Geometry: final body of the model. Coordinates: model frame, mm. Face numbers are marked on the shaded views. A direction names the side the tool comes from. Give positions to 0.01 mm unless a question says otherwise; leave off trailing zeros. Loops run counter-clockwise (first coordinate to the right, second up) from the corner with the lowest first, then second, coordinate; pieces in that order, holes last. Notation, with made-up numbers: (34.25, 46) - (79.25, 46) arc R35 cw to (79.25, 81) - close; hole circle Ø2 at (36, 24.25). An arc over 180 degrees is marked (long way). Use CSV: the item, a comma, the result in double quotes. Start each with the question number.
```python
from build123d import *

# Parameters (mm, degrees)
SKETCH1_W               = 20
SKETCH1_H               = 50
BOSS_EXTRUDE2_DEPTH     = 62.3
CUT_EXTRUDE1_DEPTH      = 1
CUT_EXTRUDE1_DEPTH_BACK = 21
BOSS_EXTRUDE3_DEPTH     = 5
SKETCH6_R               = 2.5
CUT_EXTRUDE2_DEPTH      = 5
SKETCH7_W               = 2
SKETCH7_H               = 17
CUT_EXTRUDE3_DEPTH      = 10


with BuildPart() as part:
    # Sketch1 → Boss-Extrude2 (new body)
    with BuildSketch(Plane(origin=(0, 0, 0), x_dir=(1, 0, 0), z_dir=(0, 1, 0))):
        with Locations((-10, 25)):
            Rectangle(SKETCH1_W, SKETCH1_H)
    extrude(amount=BOSS_EXTRUDE2_DEPTH)

    # Sketch2 → Cut-Extrude1 (cut, two sides)
    with BuildSketch(Plane(origin=(0, 0, 0), x_dir=(0, 0, -1), z_dir=(1, 0, 0))) as cut_extrude1_sk:
        Polygon((0, 52.3), (35.936038969, 52.3), (42.3, 45.936038969), (42.3, 16.363961031), (35.936038969, 10), (0, 10), align=None)
    extrude(amount=CUT_EXTRUDE1_DEPTH, mode=Mode.SUBTRACT)
    extrude(cut_extrude1_sk.sketch, amount=-CUT_EXTRUDE1_DEPTH_BACK, mode=Mode.SUBTRACT)

    # Sketch5 → Boss-Extrude3 (add)
    with BuildSketch(Plane.XY):
        with BuildLine():
            Line((-20, 62.3), (0, 62.3))
            ThreePointArc((0, 62.3), (-10, 72.3), (-20, 62.3))
        make_face()
        with BuildLine():
            Line((-20, 0), (0, 0))
            ThreePointArc((0, 0), (-10, -10), (-20, 0))
        make_face()
    extrude(amount=-BOSS_EXTRUDE3_DEPTH)

    # Sketch6 → Cut-Extrude2 (cut)
    with BuildSketch(Plane(origin=(0, 0, -5), x_dir=(-1, 0, 0), z_dir=(0, 0, -1))):
        with Locations((10, 66.05)):
            Circle(SKETCH6_R)
        with Locations((10, -3.75)):
            Circle(SKETCH6_R)
    extrude(amount=-CUT_EXTRUDE2_DEPTH, mode=Mode.SUBTRACT)

    # Sketch7 → Cut-Extrude3 (cut)
    with BuildSketch(Plane(origin=(0, 0, -50), x_dir=(-1, 0, 0), z_dir=(0, 0, -1))):
        with Locations((1, 31.15)):
            Rectangle(SKETCH7_W, SKETCH7_H)
    extrude(amount=-CUT_EXTRUDE3_DEPTH, mode=Mode.SUBTRACT)


solid = part.part
```
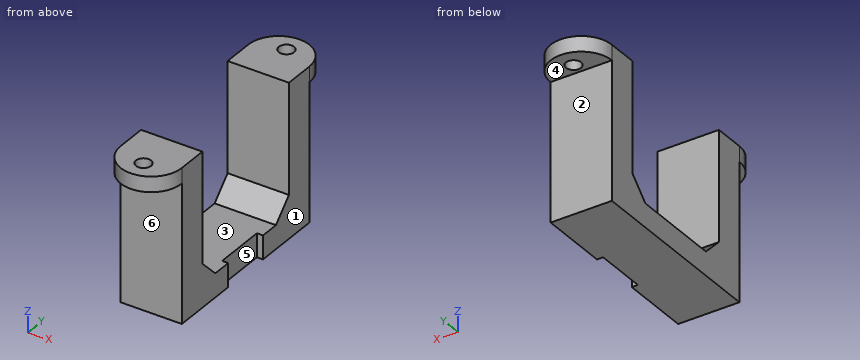
Item 1: Section D-D (z = -43.5). Output: boundary loops of the cut face in (x, y).
Item 2: Ray query, probe 1 along Y at (x, z) = (-10, -2.5); probe 2 along Y at (x, z) = (-16, -29.5); probe 3 along Y at (x, z) = (-14, -39). Return the intervals inside material, ascending.
Item 3: Section B-B (z = -15). Output: boundary loops of the cut face in (x, y), plus the area to 3 significant figures.
Item 4: Section C-C (y = 66.05). Output: boundary loops of the cut face in (x, z), plus the area to 3 significant figures.
Item 5: Section A-A (x = -11.25). Output: boundary loops of the cut face in (y, z), plus the area to 3 significant figures.
Item 6: Mould query, pull axis Y, two halves, no side actions, for the marked faces 1, 2 and 3. Classes: pulls with the +Y half, pulls with the -Y half, needs draft (parallel to the pull), parting line crosses it, or undercut.
Item 7: Reachability of the marked faces 4, 5 and 6 from +Z, -Z, +X, -X, +Y, -Y: full face, straight path, thin tool, end or side. Return the list, or none.
Item 8: Pin query (flat end, axial travel): pin 1 Ø10 at (y, z) = (60.5, -21) entering from +X; pin 2 Ø11 at (x, y) = (-14, 69.5) entering from -Z; pin 3 Ø10 at (x, z) = (-11.5, -12) entering from +Y; pin 4 Ø10 at (x, y) = (-7, 36.5) entering from +Z. Return the tip coordinate at first contact, or that it passes through.
Outcome:
1,outline,"(-20, 0) - (0, 0) - (0, 22.65) - (-2, 22.65) - (-2, 39.65) - (0, 39.65) - (0, 62.3) - (-20, 62.3) - close"
2,probe 1,"y = -10 to -6.25, -1.25 to 10, 52.3 to 63.55, 68.55 to 72.3"
2,probe 2,"y = 0 to 10, 52.3 to 62.3"
2,probe 3,"y = 0 to 13.06, 49.24 to 62.3"
3,outline,"(-20, 0) - (0, 0) - (0, 10) - (-20, 10) - close; (-20, 52.3) - (0, 52.3) - (0, 62.3) - (-20, 62.3) - close"
3,area,"400 mm2"
4,outline,"(-19.27, -5) - (-12.5, -5) - (-12.5, 0) - (-19.27, 0) - close; (-7.5, -5) - (-0.73, -5) - (-0.73, 0) - (-7.5, 0) - close"
4,area,"67.7 mm2"
5,outline,"(-9.92, -5) - (-5.92, -5) - (-5.92, 0) - (-9.92, 0) - close; (-1.58, -5) - (0, -5) - (0, -50) - (62.3, -50) - (62.3, -5) - (63.88, -5) - (63.88, 0) - (52.3, 0) - (52.3, -35.94) - (45.94, -42.3) - (16.36, -42.3) - (10, -35.94) - (10, 0) - (-1.58, 0) - close; (68.22, -5) - (72.22, -5) - (72.22, 0) - (68.22, 0) - close"
5,area,"1,420 mm2"
6,face 1,"needs draft"
6,face 2,"pulls with the +Y half"
6,face 3,"undercut"
7,face 4,"-Z, +X, -X, +Y"
7,face 5,"+Z, -Z, +X"
7,face 6,"-Z, +X, -X, -Y"
8,pin 1,"stops at x = 0"
8,pin 2,"stops at z = -5"
8,pin 3,"stops at y = 62.3"
8,pin 4,"stops at z = -42.3"
